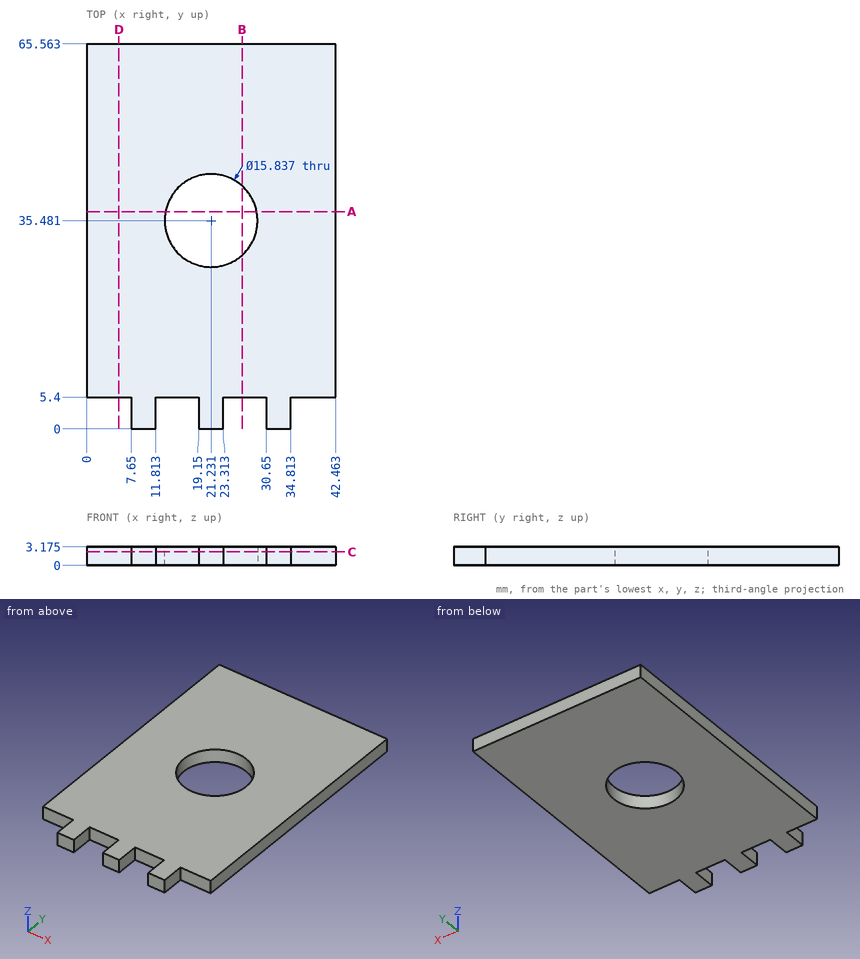
Design review of the part shown in the three views and the two pictorial views. Dimensions are in mm from the part's minimum x, y and z. Coordinates: 2 decimals unless noted, no trailing zeros. Order: outer loops, then holes, each group sorted by start corner. A loop starts at its lowest first (then second) coordinate and runs counter-clockwise, first axis right, second up. Notation, with made-up numbers: (-7, 84) -> (4, 84) arc R18 cw to (4, 109) -> close; hole circle Ø4 at (82.5, -0.75). An arc over 180 degrees is marked (long way). Use one line per item in the form item = value. Start each with the question number.
(1) Add section C-C on z = 2.3. State the section outline as (x, y) points.
(2) Insertion check: pin 1 (1.6 mm diameter, centred on y = 2.5, z = 2, fed in from +X); pin 2 (1 mm diameter, centred on x = 5.5, z = 1, fed in from -Y); pin 3 (1 mm diameter, centred on y = 3, z = 2, fed in from -X). Each pin has a flat end and moves straight along its axis. Give the tip position at first contact, or say it passes through.
(3) Add section A-A on y = 37. State the section outline as (x, z) points (1 decimal).
(4) Add section D-D on x = 5.5. State the section outline as (y, z) points (1 decimal), plus the area to 3 significant figures.
(5) Add section B-B on x = 26.5. State the section outline as (y, z) points (1 decimal).
(6) For probe 1 along Y at (x, z) = (36.5, 1.75); probe 2 along Y at (x, z) = (28.5, 2.75) (1 decimal); probe 3 along X at (y, z) = (42, 1) (1 decimal), list the stretches that pass through material, from the lowest coordinate up.
Answer block:
q1.outline = (0, 5.4) -> (7.65, 5.4) -> (7.65, 0) -> (11.81, 0) -> (11.81, 5.4) -> (19.15, 5.4) -> (19.15, 0) -> (23.31, 0) -> (23.31, 5.4) -> (30.65, 5.4) -> (30.65, 0) -> (34.81, 0) -> (34.81, 5.4) -> (42.46, 5.4) -> (42.46, 65.56) -> (0, 65.56) -> close; hole circle Ø15.84 at (21.23, 35.48)
q2.pin_1 = 34.81
q2.pin_2 = 5.4
q2.pin_3 = 7.65
q3.outline = (0, 0) -> (13.5, 0) -> (13.5, 3.2) -> (0, 3.2) -> close; (29, 0) -> (42.5, 0) -> (42.5, 3.2) -> (29, 3.2) -> close
q4.outline = (5.4, 0) -> (65.6, 0) -> (65.6, 3.2) -> (5.4, 3.2) -> close
q4.area = 191 mm²
q5.outline = (5.4, 0) -> (29.6, 0) -> (29.6, 3.2) -> (5.4, 3.2) -> close; (41.4, 0) -> (65.6, 0) -> (65.6, 3.2) -> (41.4, 3.2) -> close
q6.probe_1 = 5.4 to 65.56
q6.probe_2 = 5.4 to 32.3, 38.6 to 65.6
q6.probe_3 = 0 to 16.7, 25.7 to 42.5
